Design review of the part built by this model. Coordinates are the model's own, in mm. A direction names the side the tool comes from. Coordinates: 2 decimals unless noted, no trailing zeros. Loops run counter-clockwise (first coordinate to the right, second up) from the corner with the lowest first, then second, coordinate; pieces in that order, holes last. Notation, with made-up numbers: M 9,9.5 L 17,9.5 A12 ccw 17,20.5 Z; hole C 87,3.25 d9. An arc over 180 degrees is marked long. Put each result on its own line as item: value. Start each with the question number.
(1) For probe 1 along X at (y, z) = (6.75, 0); probe 2 along Z at (x, y) = (2.5, 8); probe 3 along Z at (x, y) = (0, 6.5), list the stretches that pass through material, from the lowest coordinate up. Write a range as [from, to].
(2) Clearance check with flat-ended pins moving along their axes: pin 1 (10 mm diameter, centred on x = 31, z = 3, fed in from -Y); pin 2 (2 mm diameter, centred on x = -0.5, z = -9.5, fed in from +Y); pin 3 (1.5 mm diameter, centred on x = 34, z = 5, fed in from -Y). State where each tip first meets the part, or that it passes through.
(3) For faces 1 (the cylindrical face through (44.1, 10.51, 4.07)), 2 (the flat face through (50, 10, 0)), 3 (the flat face through (-5, 10, -5)), 4 (the cylindrical face through (-4.07, 10.51, -10.4)), list the 3-axis set-ups (+Z, -Z, +X, -X, +Y, -Y) from which the entire face can be reached by the end or side of a thin tool; tool diameter is ignored.
(4) Take a section at C-C, the plane y = 1.5. Give the boundary of the cut face in (x, z).
(5) Take a section at D-D, the plane x = 34.5. Give the boundary of the cut face in (y, z), then the cut area to 3 significant figures.
(6) Take a section at B-B, the plane x = 20. Give the boundary of the cut face in (y, z), then the cut area to 3 significant figures.
(7) Take a section at A-A, the plane z = 0. Give the boundary of the cut face in (x, y).
```python
from build123d import *

# Parameters (mm, degrees)
SKETCH1_W           = 62
SKETCH1_H           = 22
SKETCH1_R           = 9
BOSS_EXTRUDE3_DEPTH = 10
BOSS_EXTRUDE4_START = 10
SKETCH3_W           = 7.5
SKETCH3_H           = 7.5
SKETCH3_W_2         = 15
BOSS_EXTRUDE4_DEPTH = 1
FILLET3_R           = 2


with BuildPart() as part:
    # Sketch1 → Boss-Extrude3 (new body)
    with BuildSketch(Plane(origin=(0, 0, 0), x_dir=(1, 0, 0), z_dir=(0, 1, 0))):
        with Locations((20, 0)):
            Rectangle(SKETCH1_W, SKETCH1_H)
        with Locations(Location((0, 0, 0), (0, 0, 270))):
            Circle(SKETCH1_R, mode=Mode.SUBTRACT)
        with Locations(Location((20, 0, 0), (0, 0, 270))):
            Circle(SKETCH1_R, mode=Mode.SUBTRACT)
        with Locations(Location((40, 0, 0), (0, 0, 270))):
            Circle(SKETCH1_R, mode=Mode.SUBTRACT)
    extrude(amount=BOSS_EXTRUDE3_DEPTH)

    # Sketch3 → Boss-Extrude4 (add)
    with BuildSketch(Plane(origin=(0, 0, 0), x_dir=(-1, 0, 0), z_dir=(0, 1, 0)).offset(BOSS_EXTRUDE4_START)):
        with Locations((7.25, 7.25)):
            Rectangle(SKETCH3_W, SKETCH3_H)
        with Locations((-10, 7.25)):
            Rectangle(SKETCH3_W_2, SKETCH3_H)
        with Locations((-30, 7.25)):
            Rectangle(SKETCH3_W_2, SKETCH3_H)
        with Locations((-47.25, -7.25)):
            Rectangle(SKETCH3_W, SKETCH3_H)
        with Locations((-47.25, 7.25)):
            Rectangle(SKETCH3_W, SKETCH3_H)
        with Locations((-30, -7.25)):
            Rectangle(SKETCH3_W_2, SKETCH3_H)
        with Locations((-10, -7.25)):
            Rectangle(SKETCH3_W_2, SKETCH3_H)
        with Locations((7.25, -7.25)):
            Rectangle(SKETCH3_W, SKETCH3_H)
    extrude(amount=BOSS_EXTRUDE4_DEPTH)

    # Fillet3
    fillet3_edges = [part.edges().sort_by_distance(p)[0] for p in [
        (37.5, 10.5, -11),
        (22.5, 10.5, -11),
        (22.5, 10.5, -3.5),
        (37.5, 10.5, -3.5),
        (2.5, 10.5, -3.5),
        (17.5, 10.5, -3.5),
        (17.5, 10.5, -11),
        (2.5, 10.5, -11),
        (-11, 10.5, -3.5),
        (-3.5, 10.5, -3.5),
        (-3.5, 10.5, -11),
        (-3.5, 10.5, 11),
        (-3.5, 10.5, 3.5),
        (-11, 10.5, 3.5),
        (17.5, 10.5, 3.5),
        (2.5, 10.5, 3.5),
        (2.5, 10.5, 11),
        (17.5, 10.5, 11),
        (43.5, 10.5, 3.5),
        (43.5, 10.5, 11),
        (51, 10.5, 3.5),
        (37.5, 10.5, 3.5),
        (22.5, 10.5, 3.5),
        (22.5, 10.5, 11),
        (37.5, 10.5, 11),
        (-11, 5.5, -11),
        (51, 5.5, -11),
        (51, 5.5, 11),
        (-11, 5.5, 11),
        (43.5, 10.5, -3.5),
        (51, 10.5, -3.5),
        (43.5, 10.5, -11),
    ]]
    fillet(fillet3_edges, radius=FILLET3_R)


solid = part.part
```
Computed values:
1. probe 1: x = [-11, -9], [9, 11], [29, 31], [49, 51]
1. probe 2: z = [-11, -8.65], [8.65, 11]
1. probe 3: z = [-11, -9], [9, 11]
2. pin 1: stops at y = 0
2. pin 2: stops at y = 10
2. pin 3: stops at y = 10
3. face 1: +Y, -Y
3. face 2: +X, +Y
3. face 3: -Y
3. face 4: -Z, +Y
4. outline: M -11,-9 A2 ccw -9,-11 L 49,-11 A2 ccw 51,-9 L 51,9 A2 ccw 49,11 L -9,11 A2 ccw -11,9 Z; hole C 0,0 d18; hole C 20,0 d18; hole C 40,0 d18
5. outline: M 0,-11 L 11,-11 L 11,-3.5 L 10,-3.5 L 10,-7.12 L 0,-7.12 Z; M 0,7.12 L 10,7.12 L 10,3.5 L 11,3.5 L 11,11 L 0,11 Z
5. area: 92.5 mm^2
6. outline: M 0,-11 L 10,-11 L 10,-9 L 0,-9 Z; M 0,9 L 10,9 L 10,11 L 0,11 Z
6. area: 40.0 mm^2
7. outline: M -11,0 L -9,0 L -9,10 L -11,10 Z; M 9,0 L 11,0 L 11,10 L 9,10 Z; M 29,0 L 31,0 L 31,10 L 29,10 Z; M 49,0 L 51,0 L 51,10 L 49,10 Z
